The figure shows three views and two pictorial views of one solid part (mm, origin at its lowest corner). Answer the questions. A direction names the side the tool comes from. Coordinates: 2 decimals unless noted, no trailing zeros. Write each loop counter-clockwise with the first axis right and the second up, starting at its lowest first coordinate (ties: lowest second). Pieces come first, ordered by that corner, then holes.
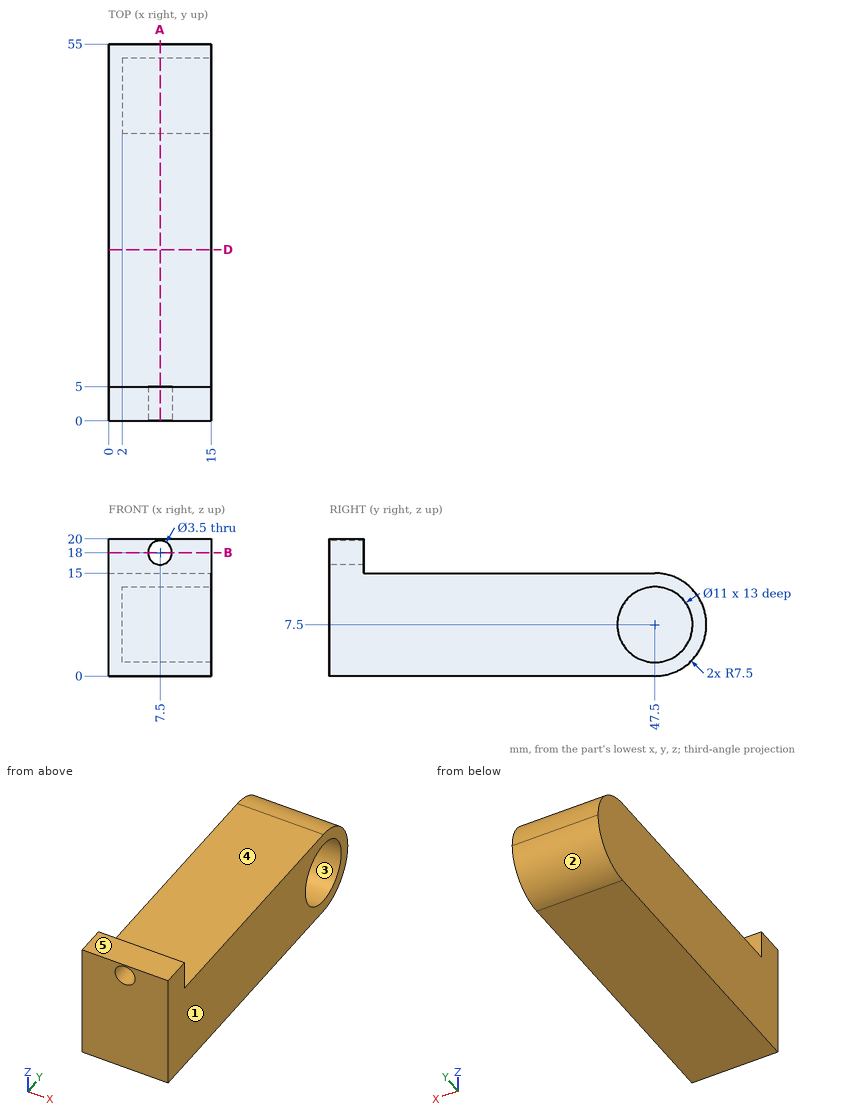
1. For a pull along Y with two mould halves and no side action, classify the marked faces 1, 2 and 3 as pulls with the +Y half, pulls with the -Y half, needs draft (parallel to the pull), parting line crosses it, or undercut.
Results found:
face 1: needs draft
face 2: pulls with the +Y half
face 3: undercut
2. A tool of negligible diameter and unlimited length cuts with its end or side. For the marked faces 4 and 5, from which of +Z, -Z, +X, -X, +Y, -Y can it reach the whole face along a straight path? Write none if from no direction.
Results found:
face 4: +Z, +X, -X, +Y
face 5: +Z, +X, -X, +Y, -Y
3. Section A-A on x = 7.5 is taken. State how many separate pieces and enclosed holes the cut face has.
Results found:
separate pieces: 2
enclosed holes: 1
4. Section D-D on y = 25 is taken. Give the vertices of the cut face in (x, z), then the cut area to 3 significant figures.
Results found:
outline: (0, 0) - (15, 0) - (15, 15) - (0, 15) - close
area: 225 mm2
5. Section B-B on z = 18 is taken. Give the vertices of the cut face in (x, y), then the cut area to 3 significant figures.
Results found:
outline: (0, 0) - (5.75, 0) - (5.75, 5) - (0, 5) - close; (9.25, 0) - (15, 0) - (15, 5) - (9.25, 5) - close
area: 57.5 mm2
6. Flat-ended cylindrical pins translate along their axes: P1, Ø4.5, axis at x = 8.5, y = 20.5, coming from the +Z side; P2, Ø4.5, axis at x = 7.5, z = 18, coming from the +Y side; P3, Ø6.5, axis at y = 47.5, z = 7.5, coming from the +X side. Find the tip coordinate at first contact, or state that the pin passes through.
Results found:
P1: stops at z = 15
P2: stops at y = 5
P3: stops at x = 2
7. Find the intervals of material crossed by L1, parallel to Y at x = 12.75, z = 7.5; L2, parallel to X at y = 3.2, z = 18; L3, parallel to Z at x = 12.5, y = 38.5, in increasing order.
Results found:
L1: y = 0 to 42, 53 to 55
L2: x = 0 to 5.75, 9.25 to 15
L3: z = 0 to 15
